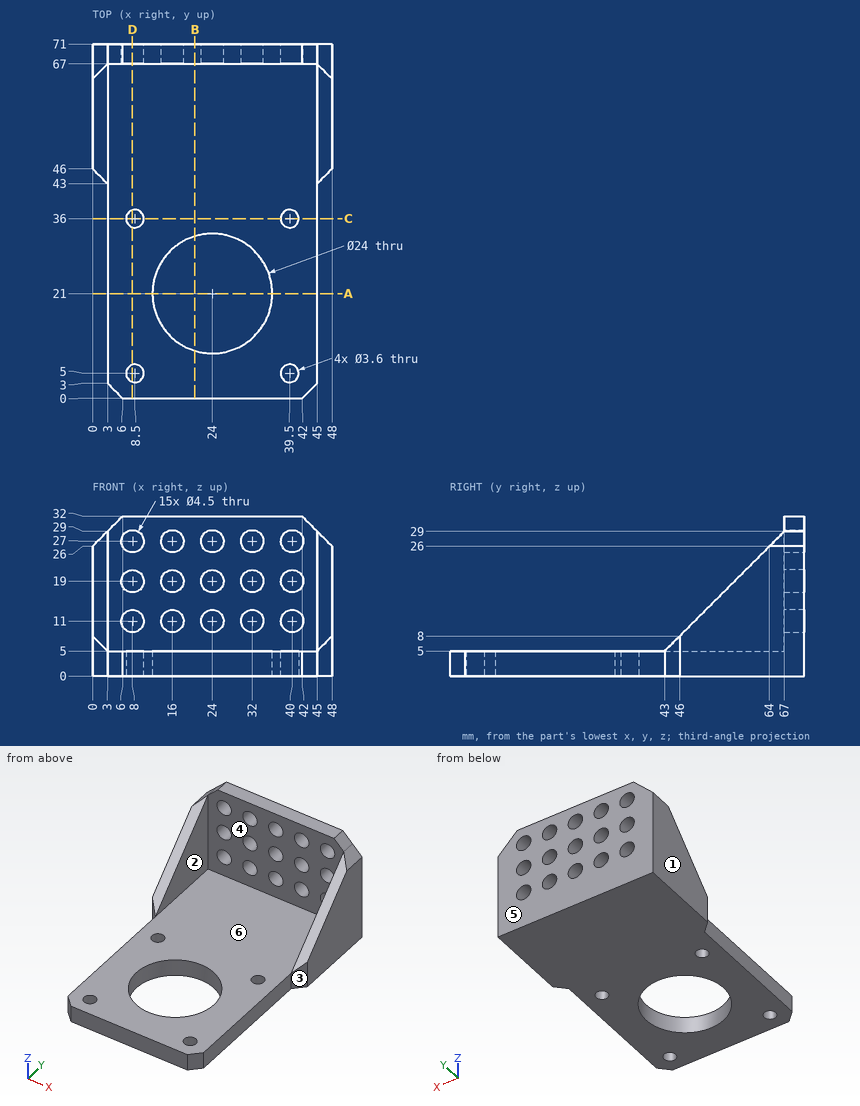
Input: dimensioned drawing with shaded views. Units: mm. Origin: part minimum x, y, z. A direction names the side the tool comes from. Give positions to 0.01 mm unless a question says otherwise; leave off trailing zeros. Write each loop counter-clockwise with the first axis right and the second up, starting at its lowest first coordinate (ties: lowest second). Pieces come first, ordered by that corner, then holes.
1. Section query D-D, the plane x = 8. Return loops of the section in (y, z).
2. Draft query along X for the marked faces 3, 4, 5 and 6. Return one class per face: released by +X, released by -X, zero draft, split by the parting line, or undercut.
3. Section query C-C, the plane y = 36. Return loops of the section in (x, z).
4. Pin query (flat end, axial travel): P1, Ø8, axis at y = 32, z = 8.5, coming from the -X side; P2, Ø6, axis at x = 35.5, y = 60.5, coming from the +Z side; P3, Ø7, axis at x = 16, z = 27, coming from the -Y side. Return the tip coordinate at first contact, or that it passes through.
5. Section query A-A, the plane y = 21. Return loops of the section in (x, z), then the cut area to 3 significant figures.
6. Section query B-B, the plane x = 20.5. Return loops of the section in (y, z), then the cut area to 3 significant figures.
7. Line query: probe 1 along X at (y, z) = (68.25, 27); probe 2 along X at (y, z) = (35.5, 4.5); probe 3 along X at (y, z) = (3.5, 2) (1 decimal). Output: solid intervals per line, ascending.
8. Reachability of the marked faces 1 and 2 from +Z, -Z, +X, -X, +Y, -Y: full face, straight path, thin tool, end or side. Return the list, or none.
Computed:
1. outline: (0, 0) - (3.27, 0) - (3.27, 5) - (0, 5) - close; (6.73, 0) - (34.27, 0) - (34.27, 5) - (6.73, 5) - close; (37.73, 0) - (71, 0) - (71, 8.75) - (67, 8.75) - (67, 5) - (37.73, 5) - close; (67, 13.25) - (71, 13.25) - (71, 16.75) - (67, 16.75) - close; (67, 21.25) - (71, 21.25) - (71, 24.75) - (67, 24.75) - close; (67, 29.25) - (71, 29.25) - (71, 32) - (67, 32) - close
2. face 3: released by +X
2. face 4: undercut
2. face 5: zero draft
2. face 6: undercut
3. outline: (3, 0) - (6.7, 0) - (6.7, 5) - (3, 5) - close; (10.3, 0) - (37.7, 0) - (37.7, 5) - (10.3, 5) - close; (41.3, 0) - (45, 0) - (45, 5) - (41.3, 5) - close
4. P1: stops at x = 3
4. P2: stops at z = 5
4. P3: stops at y = 67
5. outline: (3, 0) - (12, 0) - (12, 5) - (3, 5) - close; (36, 0) - (45, 0) - (45, 5) - (36, 5) - close
5. area: 90.0 mm2
6. outline: (0, 0) - (9.52, 0) - (9.52, 5) - (0, 5) - close; (32.48, 0) - (71, 0) - (71, 32) - (67, 32) - (67, 5) - (32.48, 5) - close
6. area: 348 mm2
7. probe 1: x = 1 to 5.75, 10.25 to 13.75, 18.25 to 21.75, 26.25 to 29.75, 34.25 to 37.75, 42.25 to 47
7. probe 2: x = 3 to 6.77, 10.23 to 37.77, 41.23 to 45
7. probe 3: x = 3 to 7.5, 9.5 to 38.5, 40.5 to 45
8. face 1: +Z, -Z, -X, +Y, -Y
8. face 2: +Z, -Y
